For this review, take the finished solid that the model builds, in its own axes (mm). Face numbers are marked on the shaded views. Round coordinates to 2 decimals unless told otherwise and drop trailing zeros. Order: outer loops, then holes, each group sorted by start corner. A loop starts at its lowest first (then second) coordinate and runs counter-clockwise, first axis right, second up. Notation, with made-up numbers: M 59.5,7 L 113.5,7 A18 ccw 113.5,30 Z; hole C 79.5,32 d3. An arc over 180 degrees is marked long. Put each result on its own line as item: value.
from build123d import *

# Parameters (mm, degrees)
SKETCH6_W          = 61.139548952
SKETCH6_H          = 56.128506874
CUT_EXTRUDE7_DEPTH = 5
SKETCH7_W          = 5
SKETCH7_H          = 10
CUT_EXTRUDE8_DEPTH = 10


with BuildPart() as part:
    # Sketch1 → Revolve1 (revolve)
    with BuildSketch(Plane.XY):
        with BuildLine():
            Line((0, 37.888888889), (0, -12.111111111))
            ThreePointArc((0, -12.111111111), (-25, 12.888888889), (0, 37.888888889))
        make_face()
    revolve(axis=Axis((0, 37.888888889, 0), (0, -1, 0)))

    # Sketch6 → Cut-Extrude7 (cut, symmetric)
    with BuildSketch(Plane(origin=(0, 0, 0), x_dir=(1, 0, 0), z_dir=(0, 1, 0))):
        Rectangle(SKETCH6_W, SKETCH6_H)
    extrude(amount=CUT_EXTRUDE7_DEPTH, both=True, mode=Mode.SUBTRACT)


with BuildPart() as body_2:
    # of the pieces the cut leaves, the one that is kept (cut_extrude7_keep)
    add(part.part.solids().sort_by_distance((-23.722677591, 5, 0))[0])

    # Sketch7 → Cut-Extrude8 (cut)
    with BuildSketch(Plane(origin=(0, 0, 0), x_dir=(1, 0, 0), z_dir=(0, 1, 0))):
        Rectangle(SKETCH7_W, SKETCH7_H)
    extrude(amount=CUT_EXTRUDE8_DEPTH, mode=Mode.SUBTRACT)


solid = body_2.part
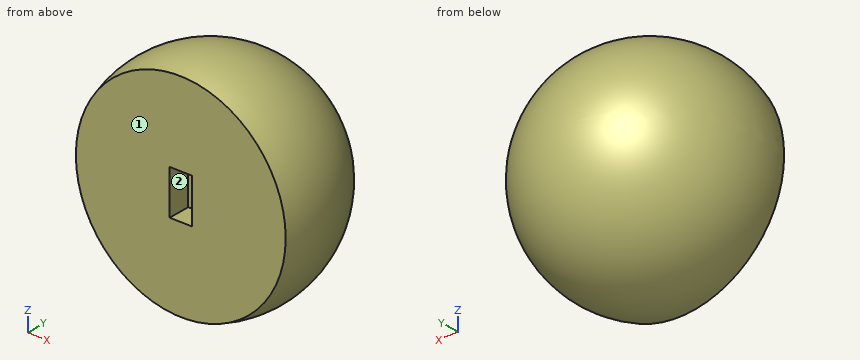
(1) Draft analysis for pull direction Z (two halves, no side actions). For the marked faces 1 and 2, state which applies: released by +Z, released by -Z, zero draft, split by the parting line, or undercut.
A:
face 1: zero draft
face 2: undercut
(2) Add section C-C on x = -17.5. Give the boundary of the cut face in (y, z).
A:
outline: M 5,-16.02 A17.85 ccw long 5,16.02 Z
(3) To check wall thickness, follow L1, parallel to Y at x = 9.5, z = -13; L2, parallel to Z at x = -5, y = 23.5; L3, parallel to Y at x = 0.5, z = -19. State the ranges of each line that lie inside material, in increasing order.
A:
L1: y = 5 to 32.01
L2: z = -22.08 to 22.08
L3: y = 5 to 29.13
(4) Add section B-B on z = 17. Give the boundary of the cut face in (x, y).
A:
outline: M -16.55,5 L 16.55,5 A18.33 ccw long Z
(5) Add section D-D on y = 12. Give the boundary of the cut face in (x, z), then the cut area to 3 significant figures.
A:
outline: C 0,0 d49.97
area: 1,960 mm2
(6) Insertion check: pin 1 Ø1.5 at (x, y) = (-1, 6.5) entering from +Z; pin 2 Ø2.5 at (x, z) = (-0.5, -1.5) entering from -Y; pin 3 Ø12 at (y, z) = (27, -18) entering from +X. Each pin has a flat end and moves straight along its axis. Give the tip position at first contact, or say it passes through.
A:
pin 1: stops at z = 24.34
pin 2: stops at y = 10
pin 3: stops at x = 18.45
(7) Add section A-A on y = 8. Give the boundary of the cut face in (x, z), then the cut area to 3 significant figures.
A:
outline: C 0,0 d49.03; hole M -2.5,-5 L 2.5,-5 L 2.5,5 L -2.5,5 Z
area: 1,840 mm2
